Model file for the job. Use its own axes, mm. Round coordinates to 2 decimals unless told otherwise and drop trailing zeros. Loops run counter-clockwise (first coordinate to the right, second up) from the corner with the lowest first, then second, coordinate; pieces in that order, holes last.
Autodesk Inventor part; units mm, degrees
ref_plane "YZ Plane" through (0, 0, 0) normal (1, 0, 0) x (0, 1, 0)
ref_plane "XZ Plane" through (0, 0, 0) normal (0, 1, 0) x (-1, 0, 0)
ref_plane "XY Plane" through (0, 0, 0) normal (0, 0, 1) x (1, 0, 0)
sketch "Sketch1" plane through (0, 0, 0) normal (0, 1, 0) x (-1, 0, 0)
  circle A0 centre (0, 0) radius 29.25
  circle A1 centre (0, 0) radius 44.25
  dimension "d0" = 58.5
  dimension "d1" = 15
extrude "Extrusion1" add sketch "Sketch1" along normal blind 40
fillet "Fillet1" radius 3 2 edges at (44.25, 40, 0) (44.25, 0, 0)
fillet "Fillet2" radius 3 2 edges at (29.25, 40, 0) (29.25, 0, 0)
properties part number "guma"
Q1. Slice it at A-A on x = 0. Give the cut face in (y, z), plus the area to 3 significant figures.
Q2. Slice it at B-B on z = 0. Give the cut face in (x, y), plus the area to 3 significant figures.
Q3. Pull direction Z, two halves, no side cores. Call faces 1 (the face through (25, 40, -21)), 2 (the face through (6.341, 19.762, 28.554)), 3 (the face through (9.59, 19.76, 43.2)): pulls with the +Z half, pulls with the -Z half, needs draft (parallel to the pull), parting line crosses it, or undercut.
Q4. Slice it at C-C on y = 9.5. Give the cut face in (x, z), plus the area to 3 significant figures.
Q5. Probe line 1 (Z direction, x = 0, y = 24); line 2 (Z direction, x = 7, y = 2); line 3 (X direction, y = 4, z = 15). List the from-to ranges inside material, lowest first.
Q6. Flat gauge pins, fed straight in: P1, Ø12, axis at y = 16, z = -34.5, coming from the +X side; P2, Ø1, axis at y = 16, z = 11.5, coming from the -X side; P3, Ø3, axis at y = 9.5, z = -24.5, coming from the +X side. Where does each tip first touch, or does it go through?
Reply:
1. outline: (0, -41.25) arc R3 ccw to (3, -44.25) - (37, -44.25) arc R3 ccw to (40, -41.25) - (40, -32.25) arc R3 ccw to (37, -29.25) - (3, -29.25) arc R3 ccw to (0, -32.25) - close; (0, 32.25) arc R3 ccw to (3, 29.25) - (37, 29.25) arc R3 ccw to (40, 32.25) - (40, 41.25) arc R3 ccw to (37, 44.25) - (3, 44.25) arc R3 ccw to (0, 41.25) - close
1. area: 1,180 mm2
2. outline: (-44.25, 3) arc R3 ccw to (-41.25, 0) - (-32.25, 0) arc R3 ccw to (-29.25, 3) - (-29.25, 37) arc R3 ccw to (-32.25, 40) - (-41.25, 40) arc R3 ccw to (-44.25, 37) - close; (29.25, 3) arc R3 ccw to (32.25, 0) - (41.25, 0) arc R3 ccw to (44.25, 3) - (44.25, 37) arc R3 ccw to (41.25, 40) - (32.25, 40) arc R3 ccw to (29.25, 37) - close
2. area: 1,180 mm2
3. face 1: needs draft
3. face 2: undercut
3. face 3: parting line crosses it
4. outline: circle Ø88.5 at (0, 0); hole circle Ø58.5 at (0, 0)
4. area: 3,460 mm2
5. line 1: z = -44.25 to -29.25, 29.25 to 44.25
5. line 2: z = -43.52 to -28.58, 28.58 to 43.52
5. line 3: x = -41.63 to -25.11, 25.11 to 41.63
6. P1: stops at x = 33.85
6. P2: stops at x = -42.86
6. P3: stops at x = 37.8
